from build123d import *

# Parameters (mm, degrees)
SKETCH1_W           = 500
SKETCH1_H           = 500
BOSS_EXTRUDE1_DEPTH = 340
SKETCH2_R           = 31
CUT_EXTRUDE1_DEPTH  = 330
SKETCH3_R           = 40
CUT_EXTRUDE3_DEPTH  = 10


with BuildPart() as part:
    # Sketch1 → Boss-Extrude1 (new body)
    with BuildSketch(Plane(origin=(0, 0, 0), x_dir=(1, 0, 0), z_dir=(0, 1, 0))):
        with Locations((200, 250)):
            Rectangle(SKETCH1_W, SKETCH1_H)
    extrude(amount=BOSS_EXTRUDE1_DEPTH)

    # Sketch2 → Cut-Extrude1 (cut)
    with BuildSketch(Plane(origin=(0, 0, 0), x_dir=(-1, 0, 0), z_dir=(0, -1, 0))):
        with Locations(Location((0, 450, 0), (0, 0, 90))):
            Circle(SKETCH2_R)
        with Locations(Location((0, 350, 0), (0, 0, 90))):
            Circle(SKETCH2_R)
        with Locations(Location((0, 250, 0), (0, 0, 90))):
            Circle(SKETCH2_R)
        with Locations(Location((0, 50, 0), (0, 0, 90))):
            Circle(SKETCH2_R)
        with Locations(Location((-100, 450, 0), (0, 0, 90))):
            Circle(SKETCH2_R)
        with Locations(Location((-100, 350, 0), (0, 0, 90))):
            Circle(SKETCH2_R)
        with Locations(Location((-100, 250, 0), (0, 0, 90))):
            Circle(SKETCH2_R)
        with Locations(Location((-100, 150, 0), (0, 0, 90))):
            Circle(SKETCH2_R)
        with Locations(Location((-100, 50, 0), (0, 0, 90))):
            Circle(SKETCH2_R)
        with Locations(Location((-200, 450, 0), (0, 0, 90))):
            Circle(SKETCH2_R)
        with Locations(Location((-200, 350, 0), (0, 0, 90))):
            Circle(SKETCH2_R)
        with Locations(Location((-200, 250, 0), (0, 0, 90))):
            Circle(SKETCH2_R)
        with Locations(Location((-200, 150, 0), (0, 0, 90))):
            Circle(SKETCH2_R)
        with Locations(Location((-200, 50, 0), (0, 0, 90))):
            Circle(SKETCH2_R)
        with Locations(Location((-300, 450, 0), (0, 0, 90))):
            Circle(SKETCH2_R)
        with Locations(Location((-300, 350, 0), (0, 0, 90))):
            Circle(SKETCH2_R)
        with Locations(Location((-300, 250, 0), (0, 0, 90))):
            Circle(SKETCH2_R)
        with Locations(Location((-300, 150, 0), (0, 0, 90))):
            Circle(SKETCH2_R)
        with Locations(Location((-300, 50, 0), (0, 0, 90))):
            Circle(SKETCH2_R)
        with Locations(Location((-400, 450, 0), (0, 0, 90))):
            Circle(SKETCH2_R)
        with Locations(Location((-400, 350, 0), (0, 0, 90))):
            Circle(SKETCH2_R)
        with Locations(Location((-400, 250, 0), (0, 0, 90))):
            Circle(SKETCH2_R)
        with Locations(Location((-400, 150, 0), (0, 0, 90))):
            Circle(SKETCH2_R)
        with Locations(Location((-400, 50, 0), (0, 0, 90))):
            Circle(SKETCH2_R)
        with Locations(Location((0, 150, 0), (0, 0, 90))):
            Circle(SKETCH2_R)
    extrude(amount=-CUT_EXTRUDE1_DEPTH, mode=Mode.SUBTRACT)

    # Sketch3 → Cut-Extrude3 (cut)
    with BuildSketch(Plane(origin=(0, 0, 0), x_dir=(-1, 0, 0), z_dir=(0, -1, 0))):
        with Locations(Location((-400, 450, 0), (0, 0, 90))):
            Circle(SKETCH3_R)
        with Locations(Location((-300, 450, 0), (0, 0, 90))):
            Circle(SKETCH3_R)
        with Locations(Location((-200, 450, 0), (0, 0, 90))):
            Circle(SKETCH3_R)
        with Locations(Location((-100, 450, 0), (0, 0, 90))):
            Circle(SKETCH3_R)
        with Locations(Location((0, 450, 0), (0, 0, 90))):
            Circle(SKETCH3_R)
        with Locations(Location((-300, 350, 0), (0, 0, 90))):
            Circle(SKETCH3_R)
        with Locations(Location((-200, 350, 0), (0, 0, 90))):
            Circle(SKETCH3_R)
        with Locations(Location((-100, 350, 0), (0, 0, 90))):
            Circle(SKETCH3_R)
        with Locations(Location((0, 350, 0), (0, 0, 90))):
            Circle(SKETCH3_R)
        with Locations(Location((-300, 250, 0), (0, 0, 90))):
            Circle(SKETCH3_R)
        with Locations(Location((-200, 250, 0), (0, 0, 90))):
            Circle(SKETCH3_R)
        with Locations(Location((-100, 250, 0), (0, 0, 90))):
            Circle(SKETCH3_R)
        with Locations(Location((0, 250, 0), (0, 0, 90))):
            Circle(SKETCH3_R)
        with Locations(Location((-300, 150, 0), (0, 0, 90))):
            Circle(SKETCH3_R)
        with Locations(Location((-200, 150, 0), (0, 0, 90))):
            Circle(SKETCH3_R)
        with Locations(Location((-100, 150, 0), (0, 0, 90))):
            Circle(SKETCH3_R)
        with Locations(Location((0, 150, 0), (0, 0, 90))):
            Circle(SKETCH3_R)
        with Locations(Location((-300, 50, 0), (0, 0, 90))):
            Circle(SKETCH3_R)
        with Locations(Location((-200, 50, 0), (0, 0, 90))):
            Circle(SKETCH3_R)
        with Locations(Location((-100, 50, 0), (0, 0, 90))):
            Circle(SKETCH3_R)
        with Locations(Location((0, 50, 0), (0, 0, 90))):
            Circle(SKETCH3_R)
        with Locations(Location((-400, 350, 0), (0, 0, 90))):
            Circle(SKETCH3_R)
        with Locations(Location((-400, 250, 0), (0, 0, 90))):
            Circle(SKETCH3_R)
        with Locations(Location((-400, 150, 0), (0, 0, 90))):
            Circle(SKETCH3_R)
        with Locations(Location((-400, 50, 0), (0, 0, 90))):
            Circle(SKETCH3_R)
    extrude(amount=-CUT_EXTRUDE3_DEPTH, mode=Mode.SUBTRACT)


solid = part.part
The listing builds one solid part. Answer for the finished solid, in the listing's coordinates (mm). Round coordinates to 2 decimals unless told otherwise and drop trailing zeros. Answer in a Markdown table with one row per item. Add a question column.
1) Determine the mould class of faces 1 (the face through (197, 340, -254)), 2 (the face through (100, 330, -250)), 3 (the face through (200, 330, -50)) for opening direction Z: pulls with the +Z half, pulls with the -Z half, needs draft (parallel to the pull), parting line crosses it, or undercut.
2) The part is cut by section A-A on y = 311. Count the separate pieces of the cut face and the enclosed holes in it, plus the area to 3 significant figures.
3) Flat-ended cylindrical pins translate along their axes: pin 1 Ø1.5 at (x, z) = (336.5, -342) entering from -Y; pin 2 Ø18.5 at (x, z) = (293.5, -144) entering from -Y. Find the tip coordinate at first contact, or state that the pin passes through.
4) Consider line 1 along X through (y, z) = (2.5, -150); line 2 along X through (y, z) = (158, -250); line 3 along Z through (x, y) = (392, 254.5). Determine where each line is inside the solid, lowest interval first. Write a range as from..to.
Findings below:
| question | item | result |
|---|---|---|
| 1 | face 1 | needs draft |
| 1 | face 2 | undercut |
| 1 | face 3 | undercut |
| 2 | separate pieces | 1 |
| 2 | enclosed holes | 25 |
| 2 | area | 175,000 mm² |
| 3 | pin 1 | stops at y = 10 |
| 3 | pin 2 | stops at y = 330 |
| 4 | line 1 | x = -50..-40, 40..60, 140..160, 240..260, 340..360, 440..450 |
| 4 | line 2 | x = -50..-31, 31..69, 131..169, 231..269, 331..369, 431..450 |
| 4 | line 3 | z = -500..-479.95, -420.05..-379.95, -320.05..-279.95, -220.05..-179.95, -120.05..-79.95, -20.05..0 |
